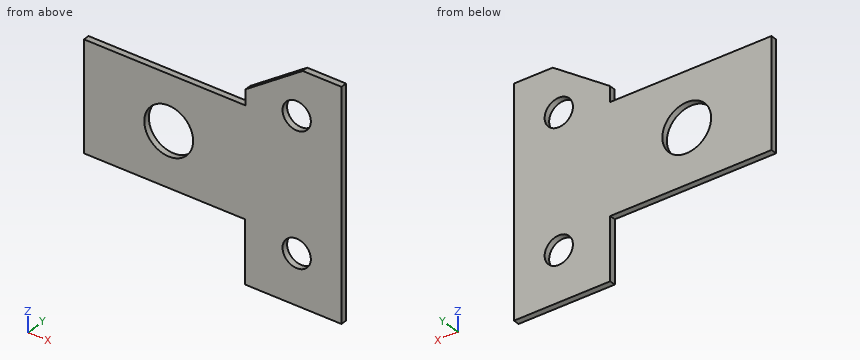
from build123d import *

# Parameters (mm, degrees)
BASE_FLANGE1_DEPTH = 1.016
SKETCH6_R          = 4.075
CUT_EXTRUDE1_DEPTH = 52.680313041
CUT_EXTRUDE2_REACH = 53.68
CUT_EXTRUDE3_REACH = 53.68
SKETCH8_R          = 2.36295848


# Sheet-metal steps are written as plain solids
with BuildPart() as part:
    # Sketch1 → Base-Flange1 (new body)
    with BuildSketch(Plane(origin=(0, 0, 0), x_dir=(1, 0, 0), z_dir=(0, 1, 0))):
        Polygon((27, 0), (27, -9.25), (43, -9.25), (43, -1.78), (43, 18.22), (43, 28.65), (26.93, 28.65), (26.93, 18.22), (0, 18.22), (0, 0), align=None)
    extrude(amount=-BASE_FLANGE1_DEPTH)

    # Sketch6 → Cut-Extrude1 (cut, through all)
    with BuildSketch(Plane(origin=(0, 0, 0), x_dir=(1, 0, 0), z_dir=(0, 1, 0))):
        with Locations(Location((14.15, 9.11, 0), (0, 0, 270))):
            Circle(SKETCH6_R)
    extrude(amount=-CUT_EXTRUDE1_DEPTH, mode=Mode.SUBTRACT)

    # Sketch7 → Cut-Extrude2 (cut, up to next)
    with BuildSketch(Plane(origin=(0, 0, 0), x_dir=(1, 0, 0), z_dir=(0, 1, 0)), mode=Mode.PRIVATE) as cut_extrude2_sk1:
        Polygon((36.522343865, -9.25), (27, -2.599722771), (27, -9.25), align=None)
    cut_extrude2_tool1 = extrude(cut_extrude2_sk1.sketch, amount=-CUT_EXTRUDE2_REACH, mode=Mode.PRIVATE) & part.part
    add(cut_extrude2_tool1.solids().sort_by_distance((30.174115, 0, 7.033241))[0], mode=Mode.SUBTRACT)

    # Sketch8 → Cut-Extrude3 (cut, up to next)
    with BuildSketch(Plane(origin=(0, 0, 0), x_dir=(1, 0, 0), z_dir=(0, 1, 0)), mode=Mode.PRIVATE) as cut_extrude3_sk1:
        with Locations(Location((35.518210435, -1.697952117, 0), (0, 0, 270))):
            Circle(SKETCH8_R)
    cut_extrude3_tool1 = extrude(cut_extrude3_sk1.sketch, amount=-CUT_EXTRUDE3_REACH, mode=Mode.PRIVATE) & part.part
    # Sketch8 → Cut-Extrude3 (cut, up to next)
    with BuildSketch(Plane(origin=(0, 0, 0), x_dir=(1, 0, 0), z_dir=(0, 1, 0)), mode=Mode.PRIVATE) as cut_extrude3_sk2:
        with Locations(Location((35.518210435, 20.302047883, 0), (0, 0, 270))):
            Circle(SKETCH8_R)
    cut_extrude3_tool2 = extrude(cut_extrude3_sk2.sketch, amount=-CUT_EXTRUDE3_REACH, mode=Mode.PRIVATE) & part.part
    add(cut_extrude3_tool1.solids().sort_by_distance((35.51821, 0, 1.697952))[0], mode=Mode.SUBTRACT)
    add(cut_extrude3_tool2.solids().sort_by_distance((35.51821, 0, -20.302048))[0], mode=Mode.SUBTRACT)


solid = part.part
The model under review builds one solid part; all positions refer to its coordinate system, in mm. Coordinates: 2 decimals unless noted, no trailing zeros. Loops run counter-clockwise (first coordinate to the right, second up) from the corner with the lowest first, then second, coordinate; pieces in that order, holes last.
(1) Wall thickness on L1, parallel to X at y = -0.75, z = -8; L2, parallel to X at y = -0.8, z = 2; L3, parallel to Z at x = 22, y = -0.65: over which ranges is each line inside the solid? List them lowest first.
Determined:
L1: x = 0 to 10.23, 18.07 to 43
L2: x = 27 to 33.17, 37.86 to 43
L3: z = -18.22 to 0
(2) Consider section B-B, the plane x = 14.15. Give the boundary of the cut face in (y, z) (3 decimals).
Determined:
outline: (-1.016, -18.22) - (0, -18.22) - (0, -13.185) - (-1.016, -13.185) - close; (-1.016, -5.035) - (0, -5.035) - (0, 0) - (-1.016, 0) - close
(3) Consider section D-D, the plane x = 31.5. Give the boundary of the cut face in (y, z).
Determined:
outline: (-1.02, -28.65) - (0, -28.65) - (0, 5.74) - (-1.02, 5.74) - close
(4) Consider section C-C, the plane y = -0.4. Give the boundary of the cut face in (x, z) (3 decimals).
Determined:
outline: (0, -18.22) - (26.93, -18.22) - (26.93, -28.65) - (43, -28.65) - (43, 9.25) - (36.522, 9.25) - (27, 2.6) - (27, 0) - (0, 0) - close; hole circle Ø8.15 at (14.15, -9.11); hole circle Ø4.726 at (35.518, -20.302); hole circle Ø4.726 at (35.518, 1.698)
(5) Insertion check: P1, Ø0.5, axis at y = -0.5, z = -24.5, coming from the -X side; P2, Ø0.5, axis at x = 12, y = -0.5, coming from the -Z side. Each pin has a flat end and moves straight along its axis. Give the tip position at first contact, or say it passes through.
Determined:
P1: stops at x = 26.93
P2: stops at z = -18.22
(6) Consider section A-A, the plane z = -9.11. Give the boundary of the cut face in (x, y) (3 decimals), plus the area to 3 significant figures.
Determined:
outline: (0, -1.016) - (10.075, -1.016) - (10.075, 0) - (0, 0) - close; (18.225, -1.016) - (43, -1.016) - (43, 0) - (18.225, 0) - close
area: 35.4 mm2
